Can you work these out from the model? Positions are in its coordinate system, mm. Face numbers are marked on the shaded views. A direction names the side the tool comes from. Coordinates: 2 decimals unless noted, no trailing zeros. Loops run counter-clockwise (first coordinate to the right, second up) from the corner with the lowest first, then second, coordinate; pieces in that order, holes last.
```python
from build123d import *

# Parameters (mm, degrees)
EXTRUDE_1_DEPTH      = 8
SKETCH_2_W           = 9
SKETCH_2_H           = 8
EXTRUDE_2_DEPTH      = 3
SKETCH_3_OUTSIDE_W   = 15.256
SKETCH_3_OUTSIDE_H   = 13.318
SKETCH_3_OUTSIDE_W_2 = 5.2
SKETCH_3_OUTSIDE_H_2 = 7
SKETCH_3_OUTSIDE_W_3 = 2
SKETCH_3_OUTSIDE_H_3 = 5
CUT_EXTRUDE_1_DEPTH  = 3.5


with BuildPart() as part:
    # 草图1 → 凸台-拉伸1 (new body)
    with BuildSketch(Plane.XY):
        Polygon((-3.062050808, 3.303627574), (-4.969401077, 0), (-2.484700538, -4.303627574), (2.484700538, -4.303627574), (4.969401077, 0), (3.062050808, 3.303627574), (1.33, 2.303627574), (2.66, 0), (1.33, -2.303627574), (-1.33, -2.303627574), (-2.66, 0), (-1.33, 2.303627574), align=None)
    extrude(amount=EXTRUDE_1_DEPTH)

    # 草图2 → 凸台-拉伸2 (add)
    with BuildSketch(Plane.XZ.offset(4.303627574)):
        with Locations((0, 4)):
            Rectangle(SKETCH_2_W, SKETCH_2_H)
    extrude(amount=EXTRUDE_2_DEPTH)

    # 草图3 outside → 切除-拉伸1 (cut)
    # profile 1 of 2: a face of its own
    with BuildSketch(Plane.XZ.offset(7.303627574)):
        with Locations((0, 4)):
            Rectangle(SKETCH_3_OUTSIDE_W, SKETCH_3_OUTSIDE_H)
        with Locations((0, 4)):
            Rectangle(SKETCH_3_OUTSIDE_W_2, SKETCH_3_OUTSIDE_H_2, mode=Mode.SUBTRACT)
    # profile 2 of 2: a face of its own
    with BuildSketch(Plane.XZ.offset(7.303627574)):
        with Locations((0, 4)):
            Rectangle(SKETCH_3_OUTSIDE_W_3, SKETCH_3_OUTSIDE_H_3)
    extrude(amount=-CUT_EXTRUDE_1_DEPTH, mode=Mode.SUBTRACT)


solid = part.part
```
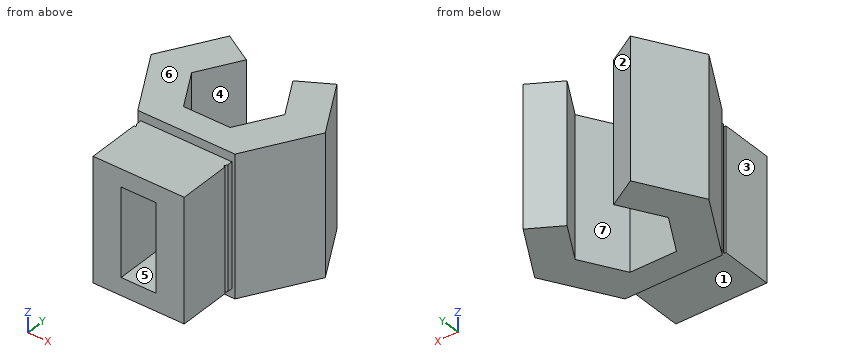
Item 1: Suppose I cut it at C-C, the plane x = 2. Please give me the cut outline in (y, z).
Results are:
outline: (-7.3, 0.5) - (-3.8, 0.5) - (-3.8, 0) - (-1.14, 0) - (-1.14, 8) - (-3.8, 8) - (-3.8, 7.5) - (-7.3, 7.5) - close; (1.14, 0) - (2.69, 0) - (2.69, 8) - (1.14, 8) - close
Item 2: I need wall thicknesses on line 1 along Z through (x, y) = (0, -4.5); line 2 along X through (y, z) = (-5.25, 4.75); line 3 along Y through (x, z) = (0.25, 3.75). Which ranges of each line are inside material? Lowest first, please.
Results are:
line 1: z = 0.5 to 1.5, 6.5 to 7.5
line 2: x = -2.6 to -1, 1 to 2.6
line 3: y = -3.8 to -2.3
Item 3: I'm going to push flat-ended pins straight in: P1, Ø1, axis at x = -4, z = 2.5, coming from the -Y side; P2, Ø1, axis at x = -0.5, y = -5.5, coming from the -Z side; P3, Ø2, axis at x = 0.5, z = 2, coming from the +Y side. Where does each tip first touch, or does it pass through?
Results are:
P1: stops at y = -2.55
P2: stops at z = 0.5
P3: stops at y = 2.4
Item 4: Suppose I cut it at B-B, the plane z = 3. Please give me the cut outline in (x, y), plus the area to 3 significant figures.
Results are:
outline: (-4.97, 0) - (-2.77, -3.8) - (-2.6, -3.8) - (-2.6, -4.1) - (-2.48, -4.3) - (-2.6, -4.3) - (-2.6, -7.3) - (-1, -7.3) - (-1, -3.8) - (1, -3.8) - (1, -7.3) - (2.6, -7.3) - (2.6, -4.3) - (2.48, -4.3) - (2.6, -4.1) - (2.6, -3.8) - (2.77, -3.8) - (4.97, 0) - (3.06, 3.3) - (1.33, 2.3) - (2.66, 0) - (1.33, -2.3) - (-1.33, -2.3) - (-2.66, 0) - (-1.33, 2.3) - (-3.06, 3.3) - close
area: 44.4 mm2
Item 5: We'd pull the mould along Z, two halves only. Please class the marked faces 5, 6 and 7: +Z half, -Z half, draft (parallel to the pull), parting line (faces both ways), or undercut.
Results are:
face 5: undercut
face 6: +Z half
face 7: draft
Item 6: Suppose I cut it at D-D, the plane y = -1.75. Please give me the cut outline in (x, z).
Results are:
outline: (-3.96, 0) - (-1.65, 0) - (-1.65, 8) - (-3.96, 8) - close; (1.65, 0) - (3.96, 0) - (3.96, 8) - (1.65, 8) - close
Item 7: On a 3-axis mill with a long thin cutter (end or side, diameter ignored), from which of +Z, -Z, +X, -X, +Y, -Y can I reach the whole of each face in a straight line? I mean the marked faces 1, 2, 3 and 4. Say none if no direction works.
Results are:
face 1: -Z, +X, -X, -Y
face 2: +Z, -Z, +Y
face 3: +Z, -Z, -X, -Y
face 4: +Z, -Z
Item 8: Suppose I cut it at A-A, the plane y = -4.75. Please give me the cut outline in (x, z), plus the area to 3 significant figures.
Results are:
outline: (-2.6, 0.5) - (2.6, 0.5) - (2.6, 7.5) - (-2.6, 7.5) - close; hole (-1, 1.5) - (1, 1.5) - (1, 6.5) - (-1, 6.5) - close
area: 26.4 mm2
